Check sheet for the modelled part. Datum: model origin and axes. Units: mm. Face numbers are marked on the shaded views. A direction names the side the tool comes from. Round coordinates to 2 decimals unless told otherwise and drop trailing zeros. Order: outer loops, then holes, each group sorted by start corner. A loop starts at its lowest first (then second) coordinate and runs counter-clockwise, first axis right, second up. Notation, with made-up numbers: (41, 5.25) -> (61, 5.25) arc R9 cw to (61, 15.25) -> close; hole circle Ø11 at (63.25, 15.25). An arc over 180 degrees is marked (long way). Answer in a Markdown table with one row per item.
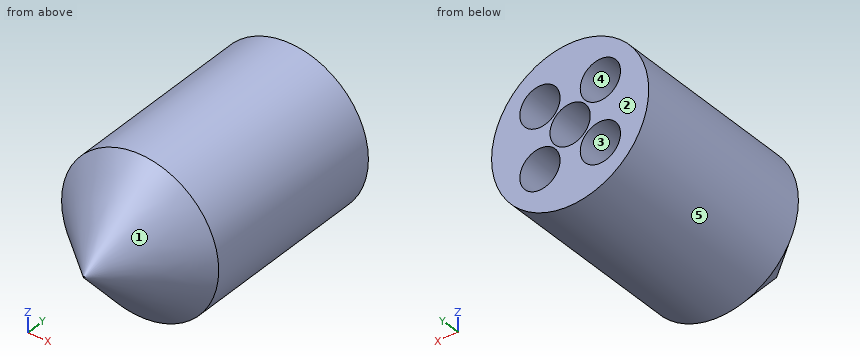
```python
from build123d import *

# Parameters (mm, degrees)
SKETCH033_R     = 9.75
PAD021_DEPTH    = 9
PAD021_TAPER    = 47
SKETCH034_R     = 9.75
PAD022_DEPTH    = 24
SKETCH035_R     = 2.5
POCKET008_DEPTH = 10


with BuildPart() as part:
    # Sketch033 → Pad021 (new body)
    with BuildSketch(Plane.XZ.offset(-20)):
        with Locations((0, -60)):
            Circle(SKETCH033_R)
    extrude(amount=PAD021_DEPTH, taper=PAD021_TAPER)

    # Sketch034 → Pad022 (join)
    with BuildSketch(Plane.XZ.offset(-20)):
        with Locations((0, -60)):
            Circle(SKETCH034_R)
    extrude(amount=-PAD022_DEPTH)

    # Sketch035 → Pocket008 (cut)
    with BuildSketch(Plane.XZ.offset(-44)):
        with Locations((-3.75, -56.25)):
            Circle(SKETCH035_R)
        with Locations((3.75, -56.25)):
            Circle(SKETCH035_R)
        with Locations((3.75, -63.75)):
            Circle(SKETCH035_R)
        with Locations((-3.75, -63.75)):
            Circle(SKETCH035_R)
        with Locations((0, -60)):
            Circle(SKETCH035_R)
    extrude(amount=POCKET008_DEPTH, mode=Mode.SUBTRACT)


solid = part.part
```
(1) Section check B-B on y = 28.5. Record the boundary of the cut face in (x, z).
Solutions:
| item | result |
|---|---|
| outline | circle Ø19.5 at (0, -60) |
(2) Section check C-C on y = 15. Record the boundary of the cut face in (x, z).
Solutions:
| item | result |
|---|---|
| outline | circle Ø8.78 at (0, -60) |
(3) Scan lines: probe 1 along Z at (x, y) = (-3.75, 40.5); probe 2 along Z at (x, y) = (0, 41); probe 3 along X at (y, z) = (35, -65.25). Record each from-to range of solid material in increasing order. Write a range as from..to.
Solutions:
| item | result |
|---|---|
| probe 1 | -69..-66.25, -61.25..-58.75, -53.75..-51 |
| probe 2 | -69.75..-62.5, -57.5..-50.25 |
| probe 3 | -8.22..-5.75, -1.75..1.75, 5.75..8.22 |
(4) Tool access check on the marked faces 4 and 5. Record the directions out of +Z, -Z, +X, -X, +Y, -Y that give a thin tool (end or side, any length) a straight path to the whole face; none if there is none.
Solutions:
| item | result |
|---|---|
| face 4 | +Y |
| face 5 | +Y, -Y |
(5) Section check A-A on y = 38. Record the boundary of the cut face in (x, z), plus the area to 3 significant figures.
Solutions:
| item | result |
|---|---|
| outline | circle Ø19.5 at (0, -60); hole circle Ø5 at (-3.75, -63.75); hole circle Ø5 at (-3.75, -56.25); hole circle Ø5 at (0, -60); hole circle Ø5 at (3.75, -63.75); hole circle Ø5 at (3.75, -56.25) |
| area | 200 mm^2 |
(6) Depth check by flat-ended pin: pin 1 Ø1.5 at (x, z) = (-3, -65) entering from +Y; pin 2 Ø4 at (x, z) = (3.75, -63.75) entering from -Y; pin 3 Ø1 at (x, y) = (-6.5, 28) entering from +Z. Enter the tip coordinate at first touch or a pass-through.
Solutions:
| item | result |
|---|---|
| pin 1 | y = 34 |
| pin 2 | y = 13.99 |
| pin 3 | z = -52.31 |
(7) Draft check along X on the marked faces 1, 2 and 3. Enter one of: pulls with the +X half, pulls with the -X half, needs draft (parallel to the pull), parting line crosses it, or undercut.
Solutions:
| item | result |
|---|---|
| face 1 | parting line crosses it |
| face 2 | needs draft |
| face 3 | undercut |
